CAD build for the part. Positions are in the model's coordinates, mm. Coordinates: 2 decimals unless noted, no trailing zeros. Write each loop counter-clockwise with the first axis right and the second up, starting at its lowest first coordinate (ties: lowest second). Pieces come first, ordered by that corner, then holes. Notation, with made-up numbers: (86.5, -8.5) - (101.5, -8.5) arc R25 cw to (101.5, 17.5) - close; hole circle Ø11 at (60, -0.5). An arc over 180 degrees is marked (long way). Answer in a Markdown table with one row per item. Add a question column.
Q1. Band-saw the part on A-A (z = 4.5). List the corners of the cut face in (x, y), and give its area (3 significant figures).
Q2. Two-plate mould, pull along X, no slides. Class faces 1 (the flat face through (0, 22, 5)), 2 (the flat face through (44, 22, 5)), 3 (the flat face through (22, 0, 5)), 4 (the cylindrical face through (12, 6, 5)): +X half, -X half, draft (parallel to the pull), parting line (faces both ways), or undercut.
Q3. Pin check, flat tip, straight feed: pin 1 (4.5 mm diameter, centred on x = 14.5, y = 38, fed in from -Z). Stop position of the tip, or through.
Q4. Band-saw the part on B-B (x = 29.5). List the corners of the cut face in (y, z), and give its area (3 significant figures).
Q5. Band-saw the part on C-C (y = 6). List the corners of the cut face in (x, z).
Q6. Drill centre lines: line 1 along Y through (x, z) = (29.5, 6.5); line 2 along X through (y, z) = (38, 3); line 3 along Y through (x, z) = (13.5, 1.25). Where is each one in solid material? Low to high. Write a range as from..to.
```python
from build123d import *

# Parameters (mm, degrees)
CYLINDER006_R     = 2.5
CYLINDER006_DEPTH = 10
CYLINDER007_R     = 2.5
CYLINDER007_DEPTH = 10
CYLINDER005_R     = 2.5
CYLINDER005_DEPTH = 10
CYLINDER004_R     = 2.5
CYLINDER004_DEPTH = 10
BOX001_W          = 44
BOX001_H          = 44
BOX001_DEPTH      = 6
CYLINDER002_R     = 2.5
CYLINDER002_DEPTH = 10
CYLINDER003_R     = 2.5
CYLINDER003_DEPTH = 10
CYLINDER001_R     = 2.5
CYLINDER001_DEPTH = 10
CYLINDER_R        = 2.5
CYLINDER_DEPTH    = 10
BOX_W             = 44
BOX_H             = 44
BOX_DEPTH         = 6


with BuildPart() as cylinder006:
    # Cylinder006 → Cylinder006 (new body)
    with BuildSketch(Plane(origin=(14.5, 38, 0), x_dir=(1, 0, 0), z_dir=(0, 0, 1))):
        Circle(CYLINDER006_R)
    extrude(amount=CYLINDER006_DEPTH)


with BuildPart() as cylinder007:
    # Cylinder007 → Cylinder007 (new body)
    with BuildSketch(Plane(origin=(29.5, 38, 0), x_dir=(1, 0, 0), z_dir=(0, 0, 1))):
        Circle(CYLINDER007_R)
    extrude(amount=CYLINDER007_DEPTH)


with BuildPart() as cylinder005:
    # Cylinder005 → Cylinder005 (new body)
    with BuildSketch(Plane(origin=(29.5, 6, 0), x_dir=(1, 0, 0), z_dir=(0, 0, 1))):
        Circle(CYLINDER005_R)
    extrude(amount=CYLINDER005_DEPTH)


with BuildPart() as cylinder004:
    # Cylinder004 → Cylinder004 (new body)
    with BuildSketch(Plane(origin=(14.5, 6, 0), x_dir=(1, 0, 0), z_dir=(0, 0, 1))):
        Circle(CYLINDER004_R)
    extrude(amount=CYLINDER004_DEPTH)


with BuildPart() as cut007:
    # Box001 → Box001 (new body)
    with BuildSketch(Plane.XY):
        with Locations((22, 22)):
            Rectangle(BOX001_W, BOX001_H)
    extrude(amount=BOX001_DEPTH)

    # Cut004: cut Cylinder004
    add(cylinder004.part, mode=Mode.SUBTRACT)

    # Cut005: cut Cylinder005
    add(cylinder005.part, mode=Mode.SUBTRACT)

    # Cut006: cut Cylinder007
    add(cylinder007.part, mode=Mode.SUBTRACT)

    # Cut007: cut Cylinder006
    add(cylinder006.part, mode=Mode.SUBTRACT)


with BuildPart() as cut007_1:
    # Cut007 placement: moved
    add(cut007.part.moved(Location((0, 0, 5))))


with BuildPart() as cylinder002:
    # Cylinder002 → Cylinder002 (new body)
    with BuildSketch(Plane(origin=(14.5, 38, 0), x_dir=(1, 0, 0), z_dir=(0, 0, 1))):
        Circle(CYLINDER002_R)
    extrude(amount=CYLINDER002_DEPTH)


with BuildPart() as cylinder003:
    # Cylinder003 → Cylinder003 (new body)
    with BuildSketch(Plane(origin=(29.5, 38, 0), x_dir=(1, 0, 0), z_dir=(0, 0, 1))):
        Circle(CYLINDER003_R)
    extrude(amount=CYLINDER003_DEPTH)


with BuildPart() as cylinder001:
    # Cylinder001 → Cylinder001 (new body)
    with BuildSketch(Plane(origin=(29.5, 6, 0), x_dir=(1, 0, 0), z_dir=(0, 0, 1))):
        Circle(CYLINDER001_R)
    extrude(amount=CYLINDER001_DEPTH)


with BuildPart() as cylinder:
    # Cylinder → Cylinder (new body)
    with BuildSketch(Plane(origin=(14.5, 6, 0), x_dir=(1, 0, 0), z_dir=(0, 0, 1))):
        Circle(CYLINDER_R)
    extrude(amount=CYLINDER_DEPTH)


with BuildPart() as fusion:
    # Box → Box (new body)
    with BuildSketch(Plane.XY):
        with Locations((22, 22)):
            Rectangle(BOX_W, BOX_H)
    extrude(amount=BOX_DEPTH)

    # Cut: cut Cylinder
    add(cylinder.part, mode=Mode.SUBTRACT)

    # Cut001: cut Cylinder001
    add(cylinder001.part, mode=Mode.SUBTRACT)

    # Cut002: cut Cylinder003
    add(cylinder003.part, mode=Mode.SUBTRACT)

    # Cut003: cut Cylinder002
    add(cylinder002.part, mode=Mode.SUBTRACT)

    # Fusion: union Cut007
    add(cut007_1.part)


solid = fusion.part
```
Checked values:
| question | item | result |
|---|---|---|
| 1 | outline | (0, 0) - (44, 0) - (44, 44) - (0, 44) - close; hole circle Ø5 at (14.5, 6); hole circle Ø5 at (14.5, 38); hole circle Ø5 at (29.5, 6); hole circle Ø5 at (29.5, 38) |
| 1 | area | 1,860 mm² |
| 2 | face 1 | -X half |
| 2 | face 2 | +X half |
| 2 | face 3 | draft |
| 2 | face 4 | undercut |
| 3 | pin 1 | passes through |
| 4 | outline | (0, 0) - (3.5, 0) - (3.5, 11) - (0, 11) - close; (8.5, 0) - (35.5, 0) - (35.5, 11) - (8.5, 11) - close; (40.5, 0) - (44, 0) - (44, 11) - (40.5, 11) - close |
| 4 | area | 374 mm² |
| 5 | outline | (0, 0) - (12, 0) - (12, 11) - (0, 11) - close; (17, 0) - (27, 0) - (27, 11) - (17, 11) - close; (32, 0) - (44, 0) - (44, 11) - (32, 11) - close |
| 6 | line 1 | y = 0..3.5, 8.5..35.5, 40.5..44 |
| 6 | line 2 | x = 0..12, 17..27, 32..44 |
| 6 | line 3 | y = 0..3.71, 8.29..35.71, 40.29..44 |
